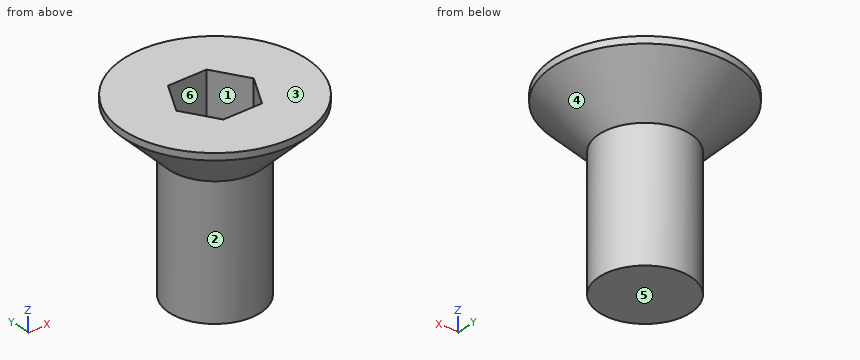
Autodesk Inventor part; units mm, degrees
ref_plane "YZ Plane" through (0, 0, 0) normal (1, 0, 0) x (0, 1, 0)
ref_plane "XZ Plane" through (0, 0, 0) normal (0, 1, 0) x (-1, 0, 0)
ref_plane "XY Plane" through (0, 0, 0) normal (0, 0, 1) x (1, 0, 0)
sketch "スケッチ1" plane through (0, 0, 0) normal (0, 0, 1) x (1, 0, 0)
  circle A0 centre (0, 0) radius 2
  dimension "d0" = 4
extrude "押し出し1" add sketch "スケッチ1" along normal blind 5.7
sketch "スケッチ2" plane through (0, 0, 5.7) normal (0, 0, 1) x (1, 0, 0)
  circle A0 centre (0, 0) radius 4
  dimension "d3" = 8
extrude "押し出し2" add sketch "スケッチ2" along normal blind 2.3
chamfer "面取り1" distance 2 angle 45 1 edges at (-4, 0, 5.7)
sketch "スケッチ3" plane through (0, 0, 8) normal (0, 0, 1) x (1, 0, 0)
  line L0 (1.7321, 0) -> (0.866, -1.5)
  line L1 (0.866, -1.5) -> (-0.866, -1.5)
  line L2 (-0.866, -1.5) -> (-1.7321, 0)
  line L3 (-1.7321, 0) -> (-0.866, 1.5)
  line L4 (-0.866, 1.5) -> (0.866, 1.5)
  line L5 (0.866, 1.5) -> (1.7321, 0)
  point P0 (0, 0)
  point P1 (0, 0)
  dimension "d9" = 3
extrude "押し出し3" cut sketch "スケッチ3" against normal blind 2
thread "ねじ1"
properties part number "M4皿ネジ　8" material "鉄 灰色"
Work out the finished part from the listing and answer in its coordinate system (mm). Face numbers are marked on the shaded views. A direction names the side the tool comes from. Coordinates: 2 decimals unless noted, no trailing zeros. Order: outer loops, then holes, each group sorted by start corner. A loop starts at its lowest first (then second) coordinate and runs counter-clockwise, first axis right, second up. Notation, with made-up numbers: (46.5, 70) - (88.5, 70) arc R17 ccw to (88.5, 99) - close; hole circle Ø4 at (89.5, 64.25). An arc over 180 degrees is marked (long way). Answer as a JSON object with one key per item and string values.
1. A tool of negligible diameter and unlimited length cuts with its end or side. For the marked faces 1, 2 and 3, from which of +Z, -Z, +X, -X, +Y, -Y can it reach the whole face along a straight path? Write none if from no direction.
Output values:
{"face 1": "+Z", "face 2": "-Z", "face 3": "+Z, +X, -X, +Y, -Y"}
2. Find section C-C on z = 4.75. Determine the outline of the cut face in (x, y).
Output values:
{"outline": "circle Ø4 at (0, 0)"}
3. The mould has two halves that part along Y. Classify the marked faces 4, 5 and 6: +Y half, -Y half, draft (parallel to the pull), parting line (faces both ways), or undercut.
Output values:
{"face 4": "parting line", "face 5": "draft", "face 6": "undercut"}
4. Each of these flat-tipped pins is pushed along its axis until it touches: P1, Ø3, axis at x = -3, z = 1, coming from the -Y side; P2, Ø0.5, axis at x = 0.5, z = 6.5, coming from the -Y side. Where does it stop, or does it pass through?
Output values:
{"P1": "stops at y = -1.32", "P2": "stops at y = -3.01"}
5. Consider line 1 (X direction, y = -0.5, z = 6.75); line 2 (Z direction, x = -0.75, y = 0.5); line 3 (Z direction, x = -3, y = -1). Determine where each line is inside the solid, lowest interval first.
Output values:
{"line 1": "x = -3.01 to -1.44, 1.44 to 3.01", "line 2": "z = 0 to 6", "line 3": "z = 6.86 to 8"}
6. Find section A-A on z = 7. Determine the outline of the cut face in (x, y).
Output values:
{"outline": "circle Ø6.6 at (0, 0); hole (-1.73, 0) - (-0.87, -1.5) - (0.87, -1.5) - (1.73, 0) - (0.87, 1.5) - (-0.87, 1.5) - close"}
